Here's how the part is built. I have some questions about the finished solid (model axes, mm). Face numbers are marked on the shaded views. A direction names the side the tool comes from. Round coordinates to 2 decimals unless told otherwise and drop trailing zeros. Loops run counter-clockwise (first coordinate to the right, second up) from the corner with the lowest first, then second, coordinate; pieces in that order, holes last. Notation, with made-up numbers: (45.25, -37.5) -> (55.25, -37.5) arc R23 ccw to (55.25, -17.5) -> close; hole circle Ø6 at (6, 39.25). An arc over 180 degrees is marked (long way). Use one line per item in the form item = value. Start each with the question number.
Item 1: If we section it at A-A (z = 0): Write out the boundary of the cut face in (x, y) (3 decimals).
Item 2: I'm going to push flat-ended pins straight in: pin 1 Ø7 at (x, z) = (9.525, 0) entering from -Y; pin 2 Ø7 at (x, z) = (-9.525, 0) entering from +Y. Where does each tip first touch, or does it pass through?
Item 3: Thinking about a two-plate mould opening in X: for the marked faces 3, 4 and 5, which applies, released by +X, released by -X, zero draft, split by the parting line, or undercut?
Item 4: For the marked faces 1 and 2, which set-ups out of +Z, -Z, +X, -X, +Y, -Y let a thin tool reach every point of the face, with its end or its side?
Item 5: If we section it at B-B (x = -17): Write out the boundary of the cut face in (y, z).
Item 6: If I drill on L1, parallel to X at y = 1.4, z = 0 (3 decimals); L2, parallel to X at y = 3, z = -3.25 (3 decimals); L3, parallel to Z at x = 21, y = 5, over which ranges is the centre line in solid material (lowest first)? Write a range as [from, to].
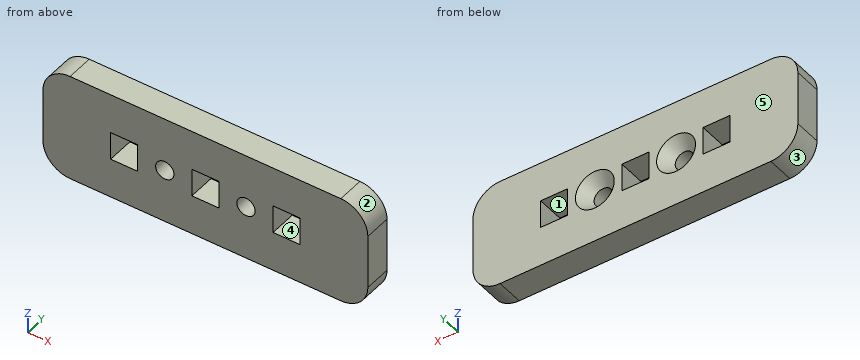
```python
from build123d import *

# Parameters (mm, degrees)
SKETCH1_W                                         = 76.2
SKETCH1_H                                         = 25.4
BOSS_EXTRUDE1_DEPTH                               = 6.35
SKETCH2_R                                         = 2.15265
SKETCH2_W                                         = 6.35
SKETCH2_H                                         = 6.604
CUT_EXTRUDE1_DEPTH                                = 7.35
FILLET1_R                                         = 6.35
CSK_FOR_8_FLAT_HEAD_SOCKET_CAP_SCREW1_D           = 4.3053
CSK_FOR_8_FLAT_HEAD_SOCKET_CAP_SCREW1_CSINK_D     = 9.1186
CSK_FOR_8_FLAT_HEAD_SOCKET_CAP_SCREW1_CSINK_ANGLE = 82


with BuildPart() as part:
    # Sketch1 → Boss-Extrude1 (new body)
    with BuildSketch(Plane(origin=(0, 0, 0), x_dir=(1, 0, 0), z_dir=(0, 1, 0))):
        Rectangle(SKETCH1_W, SKETCH1_H)
    extrude(amount=BOSS_EXTRUDE1_DEPTH)

    # Sketch2 → Cut-Extrude1 (cut, through all)
    with BuildSketch(Plane(origin=(0, 6.35, 0), x_dir=(1, 0, 0), z_dir=(0, 1, 0))):
        with Locations((-9.525, 0)):
            Circle(SKETCH2_R)
        with Locations((9.525, 0)):
            Circle(SKETCH2_R)
        Rectangle(SKETCH2_W, SKETCH2_H)
        with Locations((-19.05, 0)):
            Rectangle(SKETCH2_W, SKETCH2_H)
        with Locations((19.05, 0)):
            Rectangle(SKETCH2_W, SKETCH2_H)
    extrude(amount=-CUT_EXTRUDE1_DEPTH, mode=Mode.SUBTRACT)

    # Fillet1
    fillet1_edges = [part.edges().sort_by_distance(p)[0] for p in [
        (-38.1, 3.175, -12.7),
        (38.1, 3.175, -12.7),
        (38.1, 3.175, 12.7),
        (-38.1, 3.175, 12.7),
    ]]
    fillet(fillet1_edges, radius=FILLET1_R)

    # CSK for #8 Flat Head Socket Cap Screw1 (through all)
    with Locations(Plane(origin=(0, 6.35, 0), x_dir=(1, 0, 0), z_dir=(0, 1, 0))):
        with Locations((-9.525, 0), (9.525, 0)):
            CounterSinkHole(CSK_FOR_8_FLAT_HEAD_SOCKET_CAP_SCREW1_D / 2, CSK_FOR_8_FLAT_HEAD_SOCKET_CAP_SCREW1_CSINK_D / 2, counter_sink_angle=CSK_FOR_8_FLAT_HEAD_SOCKET_CAP_SCREW1_CSINK_ANGLE)


solid = part.part
```
Values found:
q1.outline = (-38.1, 0) -> (-22.225, 0) -> (-22.225, 6.35) -> (-38.1, 6.35) -> close; (-15.875, 0) -> (-11.678, 0) -> (-11.678, 3.581) -> (-14.084, 6.35) -> (-15.875, 6.35) -> close; (-7.372, 0) -> (-3.175, 0) -> (-3.175, 6.35) -> (-4.966, 6.35) -> (-7.372, 3.581) -> close; (3.175, 0) -> (7.372, 0) -> (7.372, 3.581) -> (4.966, 6.35) -> (3.175, 6.35) -> close; (11.678, 0) -> (15.875, 0) -> (15.875, 6.35) -> (14.084, 6.35) -> (11.678, 3.581) -> close; (22.225, 0) -> (38.1, 0) -> (38.1, 6.35) -> (22.225, 6.35) -> close
q2.pin_1 = 0
q2.pin_2 = 5.13
q3.face_3 = released by -X
q3.face_4 = undercut
q3.face_5 = zero draft
q4.face_1 = +Y, -Y
q4.face_2 = +Z, +X, +Y, -Y
q5.outline = (0, -12.7) -> (6.35, -12.7) -> (6.35, -3.3) -> (0, -3.3) -> close; (0, 3.3) -> (6.35, 3.3) -> (6.35, 12.7) -> (0, 12.7) -> close
q6.L1 = [-38.1, -22.225], [-15.875, -11.678], [-7.372, -3.175], [3.175, 7.372], [11.678, 15.875], [22.225, 38.1]
q6.L2 = [-38.1, -22.225], [-15.875, -3.175], [3.175, 15.875], [22.225, 38.1]
q6.L3 = [-12.7, -3.3], [3.3, 12.7]
